Work out the finished part from the listing and answer in its coordinate system (mm). A direction names the side the tool comes from. Round coordinates to 2 decimals unless told otherwise and drop trailing zeros. Loops run counter-clockwise (first coordinate to the right, second up) from the corner with the lowest first, then second, coordinate; pieces in that order, holes last.
```python
from build123d import *

# Parameters (mm, degrees)
SKETCH_1_W          = 70
SKETCH_1_H          = 80
EXTRUDE_1_DEPTH     = 3
SKETCH_4_R          = 2.1
SKETCH_4_W          = 40.676852231
SKETCH_4_H          = 20.906984827
CUT_EXTRUDE_3_DEPTH = 10
SKETCH_5_R          = 1.5
CUT_EXTRUDE_4_DEPTH = 10
FILLET_1_R          = 10


with BuildPart() as part:
    # 草图1 → 凸台-拉伸1 (new body)
    with BuildSketch(Plane.XY):
        Rectangle(SKETCH_1_W, SKETCH_1_H)
    extrude(amount=EXTRUDE_1_DEPTH)

    # 草图4 → 切除-拉伸3 (cut)
    with BuildSketch(Plane(origin=(0, 0, 0), x_dir=(-1, 0, 0), z_dir=(0, 0, -1))):
        with Locations((24.25, -14.575)):
            Circle(SKETCH_4_R)
        with Locations((24.25, -5.075)):
            Circle(SKETCH_4_R)
        with Locations((-24.25, -14.575)):
            Circle(SKETCH_4_R)
        with Locations((-24.25, -5.075)):
            Circle(SKETCH_4_R)
        with Locations((0.054839574, -10.049357678)):
            Rectangle(SKETCH_4_W, SKETCH_4_H)
    extrude(amount=-CUT_EXTRUDE_3_DEPTH, mode=Mode.SUBTRACT)

    # 草图5 → 切除-拉伸4 (cut)
    with BuildSketch(Plane.XY.offset(3)):
        with Locations((-20, 30)):
            Circle(SKETCH_5_R)
        with Locations((0, 30)):
            Circle(SKETCH_5_R)
        with Locations((20, 30)):
            Circle(SKETCH_5_R)
    extrude(amount=-CUT_EXTRUDE_4_DEPTH, mode=Mode.SUBTRACT)

    # 圆角1
    fillet_1_edges = [part.edges().sort_by_distance(p)[0] for p in [
        (35, -40, 1.5),
        (-35, -40, 1.5),
        (-35, 40, 1.5),
        (35, 40, 1.5),
    ]]
    fillet(fillet_1_edges, radius=FILLET_1_R)


solid = part.part
```
1. Find section C-C (z = 1.45). Give the number of separate pieces and of enclosed holes in the cut face, then the cut area to 3 significant figures.
Answer key:
separate pieces: 1
enclosed holes: 8
area: 4,590 mm2
2. Which of the six approach directions +Z, -Z, +X, -X, +Y, -Y give full straight-line access (tool end or side, diameter ignored) to faces 1 (the face through (35, 0, 1)), 2 (the face through (0, 0.404, 1))?
Answer key:
face 1: +Z, -Z, +X, +Y, -Y
face 2: +Z, -Z
3. Find section B-B (x = 0). Write down the section's boundary in (y, z).
Answer key:
outline: (-40, 0) - (-20.5, 0) - (-20.5, 3) - (-40, 3) - close; (0.4, 0) - (28.5, 0) - (28.5, 3) - (0.4, 3) - close; (31.5, 0) - (40, 0) - (40, 3) - (31.5, 3) - close
4. Find section A-A (x = -15). Write down the section's boundary in (y, z), then the cut area to 3 significant figures.
Answer key:
outline: (-40, 0) - (-20.5, 0) - (-20.5, 3) - (-40, 3) - close; (0.4, 0) - (40, 0) - (40, 3) - (0.4, 3) - close
area: 177 mm2
5. Consider probe 1 along Y at (x, z) = (0, 2.25); probe 2 along X at (y, z) = (-17, 0.85); probe 3 along Y at (x, z) = (-11, 1.5). Determine where each line is inside the solid, lowest interval first.
Answer key:
probe 1: y = -40 to -20.5, 0.4 to 28.5, 31.5 to 40
probe 2: x = -35 to -20.39, 20.28 to 35
probe 3: y = -40 to -20.5, 0.4 to 40
6. Determine the mould class of faces 3 (the face through (-32.15, 36.99, 1.52)), 4 (the face through (-20.393, -10, 1)), 5 (the face through (-26.25, -13.94, 1.48)), 6 (the face through (0, 1, 3)) for opening direction Y: +Y half, -Y half, draft (parallel to the pull), parting line (faces both ways), or undercut.
Answer key:
face 3: +Y half
face 4: undercut
face 5: undercut
face 6: draft
7. Given pin 1 (1 mm diameter, centred on x = -8.5, y = 2.5, fed in from -Z); pin 2 (4 mm diameter, centred on x = -24.25, y = -14.575, fed in from -Z), each flat-ended and moving along its own axis, determine where each tip first touches the part or whether it passes through.
Answer key:
pin 1: stops at z = 0
pin 2: passes through
